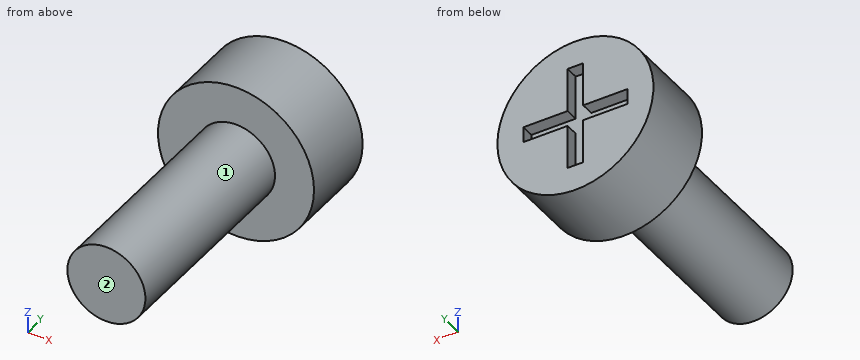
Autodesk Inventor part; units mm, degrees
ref_plane "YZ Plane" through (0, 0, 0) normal (1, 0, 0) x (0, 1, 0)
ref_plane "XZ Plane" through (0, 0, 0) normal (0, 1, 0) x (-1, 0, 0)
ref_plane "XY Plane" through (0, 0, 0) normal (0, 0, 1) x (1, 0, 0)
sketch "Sketch1" plane through (0, 0, 0) normal (0, 1, 0) x (-1, 0, 0)
  circle A0 centre (0, 0) radius 1.5
  dimension "d0" = 3
extrude "Extrusion1" add sketch "Sketch1" along normal blind 8
sketch "Sketch2" plane through (0, 8, 0) normal (0, 1, 0) x (1, 0, 0)
  circle A0 centre (0, 0) radius 3
  dimension "d3" = 6
extrude "Extrusion2" add sketch "Sketch2" along normal blind 3
sketch "Sketch3" plane through (0, 11, 0) normal (0, 1, 0) x (1, 0, 0)
  line L0 (-2, -0.3) -> (-0.3, -0.3)
  line L1 (-0.3, -0.3) -> (-0.3, -2)
  line L2 (-0.3, -2) -> (0.3, -2)
  line L3 (0.3, -2) -> (0.3, -0.3)
  line L4 (0.3, -0.3) -> (2, -0.3)
  line L5 (2, -0.3) -> (2, 0.3)
  line L6 (2, 0.3) -> (0.3, 0.3)
  line L7 (0.3, 0.3) -> (0.3, 2)
  line L8 (0.3, 2) -> (-0.3, 2)
  line L9 (-0.3, 2) -> (-0.3, 0.3)
  line L10 (-2, 0.3) -> (-2, -0.3)
  line L11 (-2, 0.3) -> (-0.3, 0.3)
  circle A0 centre (0, 0) radius 3
  point P0 (0, 0)
  dimension "d19" = 0.3
  dimension "d20" = 0.3
  dimension "d22" = 2
  dimension "d23" = 0
  dimension "d26" = 0.3
  dimension "d27" = 0.3
extrude "Extrusion3" cut sketch "Sketch3" against normal blind 0.5 contours L10 L11 L9 L8 L7 L6 L5 L4 L3 L2 L1 L0
thread "Thread1"
properties part number "BoltM3-PI" material "PC/ABS Plastic"
Could you check a few things on this model? Use its own coordinates, in mm. Face numbers are marked on the shaded views. A direction names the side the tool comes from. Coordinates: 2 decimals unless noted, no trailing zeros. Loops run counter-clockwise (first coordinate to the right, second up) from the corner with the lowest first, then second, coordinate; pieces in that order, holes last.
1) Imagine slicing it at B-B (z = 0). List the corners of the cut face in (x, y) for me, and give its area (3 significant figures).
Reported:
outline: (-3, 8) - (-1.5, 8) - (-1.5, 0) - (1.5, 0) - (1.5, 8) - (3, 8) - (3, 11) - (2, 11) - (2, 10.5) - (-2, 10.5) - (-2, 11) - (-3, 11) - close
area: 40.0 mm2
2) Imagine slicing it at C-C (y = 2.5). List the corners of the cut face in (x, z) for me, and give its area (3 significant figures).
Reported:
outline: circle Ø3 at (0, 0)
area: 7.07 mm2
3) Please list where these lines run through material, in increasing order: line 1 along Y through (x, z) = (1.1, 2.25); line 2 along Y through (x, z) = (0.25, -0.1); line 3 along X through (y, z) = (8.5, -1.7).
Reported:
line 1: y = 8 to 11
line 2: y = 0 to 10.5
line 3: x = -2.47 to 2.47
4) Imagine slicing it at D-D (x = 1.75). List the corners of the cut face in (y, z) for me, and give its area (3 significant figures).
Reported:
outline: (8, -2.44) - (11, -2.44) - (11, -0.3) - (10.5, -0.3) - (10.5, 0.3) - (11, 0.3) - (11, 2.44) - (8, 2.44) - close
area: 14.3 mm2
5) Will these pins go through, and if not, where does the flat tip stop? pin 1 Ø1 at (y, z) = (9.5, 2) entering from +X; pin 2 Ø2 at (y, z) = (1.5, -1.5) entering from -X; pin 3 Ø0.6 at (y, z) = (10.5, -1) entering from +X.
Reported:
pin 1: stops at x = 2.6
pin 2: stops at x = -1.41
pin 3: stops at x = 2.92
6) Which directions (+Z, -Z, +X, -X, +Y, -Y) give clear straight access to the entire face, cutting with the end or side of a thin tool? Please do the marked faces 1 and 2.
Reported:
face 1: -Y
face 2: +Z, -Z, +X, -X, -Y
7) Imagine slicing it at A-A (x = 0). List the corners of the cut face in (y, z) for me.
Reported:
outline: (0, -1.5) - (8, -1.5) - (8, -3) - (11, -3) - (11, -2) - (10.5, -2) - (10.5, 2) - (11, 2) - (11, 3) - (8, 3) - (8, 1.5) - (0, 1.5) - close
